Geometry check sheet. Reference: the model listing, model coordinates, mm. Face numbers are marked on the shaded views. Coordinates: 2 decimals unless noted, no trailing zeros. Write each loop counter-clockwise with the first axis right and the second up, starting at its lowest first coordinate (ties: lowest second). Pieces come first, ordered by that corner, then holes. Notation, with made-up numbers: (21.5, 15.5) -> (30.5, 15.5) arc R22 cw to (30.5, 49.5) -> close; hole circle Ø7 at (29.25, -22). An arc over 180 degrees is marked (long way). One line per question, with ' | ' between items.
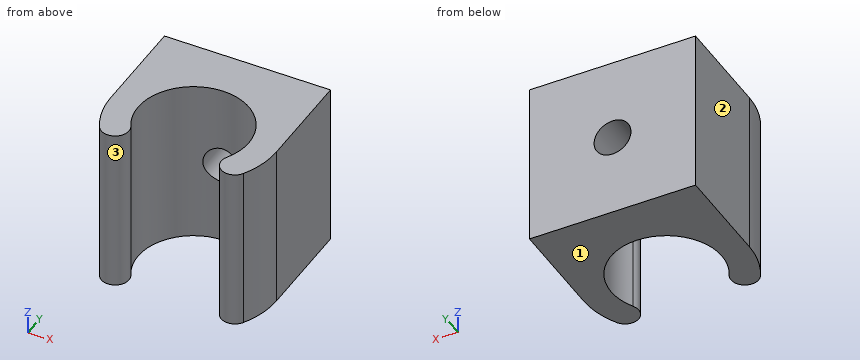
```python
from build123d import *

# Parameters (mm, degrees)
AUFSATZ_LINEAR_AUSTRAGEN1_DEPTH      = 4.5
SCHNITT_LINEAR_AUSTRAGEN1_REACH      = 12.317
SCHNITT_LINEAR_AUSTRAGEN1_END_RADIUS = 3
SKIZZE3_R                            = 1


with BuildPart() as part:
    # Skizze1 → Aufsatz-Linear austragen1 (new, symmetric)
    with BuildSketch(Plane.XY):
        with BuildLine():
            Line((-4.5, 5.5), (4.5, 5.5))
            Line((4.5, 5.5), (4.5, 0))
            ThreePointArc((4.5, 0), (4.347413024, -1.161895004), (3.9, -2.244994432))
            ThreePointArc((3.9, -2.244994432), (2.875834261, -2.520828693), (2.6, -1.496662955))
            ThreePointArc((2.6, -1.496662955), (0, 3), (-2.6, -1.496662955))
            ThreePointArc((-2.6, -1.496662955), (-2.875834261, -2.520828693), (-3.9, -2.244994432))
            ThreePointArc((-3.9, -2.244994432), (-4.347413024, -1.161895004), (-4.5, 0))
            Line((-4.5, 0), (-4.5, 5.5))
        make_face()
    extrude(amount=AUFSATZ_LINEAR_AUSTRAGEN1_DEPTH, both=True)

    # Schnitt-Linear austragen1: up to this cylinder (the profile starts outside it)
    schnitt_linear_austragen1_end = Plane(origin=(0, 0, 0), z_dir=(0, 0, -1)) * Cylinder(SCHNITT_LINEAR_AUSTRAGEN1_END_RADIUS, 31.634, mode=Mode.PRIVATE)
    # Skizze3 → Schnitt-Linear austragen1 (cut, up to the surface)
    with BuildSketch(Plane(origin=(0, 5.5, 0), x_dir=(1, 0, 0), z_dir=(0, 1, 0)), mode=Mode.PRIVATE) as schnitt_linear_austragen1_sk1:
        with Locations(Location((0, 0, 0), (0, 0, 270))):
            Circle(SKIZZE3_R)
    schnitt_linear_austragen1_tool1 = extrude(schnitt_linear_austragen1_sk1.sketch, amount=-SCHNITT_LINEAR_AUSTRAGEN1_REACH, mode=Mode.PRIVATE) - schnitt_linear_austragen1_end
    add(schnitt_linear_austragen1_tool1.solids().sort_by_distance((0, 5.5, 0))[0], mode=Mode.SUBTRACT)


solid = part.part
```
(1) Cross-section at C-C (y = 5.25). Record the cut outline in (x, z).
Answers below:
outline: (-4.5, -4.5) -> (4.5, -4.5) -> (4.5, 4.5) -> (-4.5, 4.5) -> close; hole circle Ø2 at (0, 0)
(2) Draft check along X on the marked faces 1, 2 and 3. Enter one of: pulls with the +X half, pulls with the -X half, needs draft (parallel to the pull), parting line crosses it, or undercut.
Answers below:
face 1: needs draft | face 2: pulls with the -X half | face 3: undercut
(3) Material ranges on line 1 (X direction, y = 4.35, z = 0); line 2 (Y direction, x = 1, z = 1.5), recorded low to high.
Answers below:
line 1: x = -4.5 to -1, 1 to 4.5 | line 2: y = 2.83 to 5.5
(4) Cross-section at A-A (x = 0). Record the cut outline in (y, z).
Answers below:
outline: (3, -4.5) -> (5.5, -4.5) -> (5.5, -1) -> (3, -1) -> close; (3, 1) -> (5.5, 1) -> (5.5, 4.5) -> (3, 4.5) -> close
(5) Depth check by flat-ended pin: P1, Ø1, axis at y = -1.5, z = 2, coming from the -X side. Enter the tip coordinate at first touch or a pass-through.
Answers below:
P1: stops at x = -4.39
(6) Cross-section at D-D (y = 1.25). Record the cut outline in (x, z), plus the area to 3 significant figures.
Answers below:
outline: (-4.5, -4.5) -> (-2.73, -4.5) -> (-2.73, 4.5) -> (-4.5, 4.5) -> close; (2.73, -4.5) -> (4.5, -4.5) -> (4.5, 4.5) -> (2.73, 4.5) -> close | area: 31.9 mm²
(7) Cross-section at B-B (z = 0). Record the cut outline in (x, y) (3 decimals).
Answers below:
outline: (-4.5, 0) arc R4.5 ccw to (-3.9, -2.245) arc R0.75 ccw to (-2.6, -1.497) arc R3 cw to (-1, 2.828) -> (-1, 5.5) -> (-4.5, 5.5) -> close; (1, 2.828) arc R3 cw to (2.6, -1.497) arc R0.75 ccw to (3.9, -2.245) arc R4.5 ccw to (4.5, 0) -> (4.5, 5.5) -> (1, 5.5) -> close
